Source: CAD feature listing. Evaluate the final solid. Frame: model axes, mm. A direction names the side the tool comes from. Round coordinates to 2 decimals unless told otherwise and drop trailing zeros. Write each loop counter-clockwise with the first axis right and the second up, starting at its lowest first coordinate (ties: lowest second). Pieces come first, ordered by that corner, then holes. Notation, with made-up numbers: M -20,-20.5 L 26,-20.5 A25 cw 26,4.5 Z; hole C 1.5,6 d4. An arc over 180 degrees is marked long. Put each result on its own line as item: value. Start each with the question number.
```python
from build123d import *

# Parameters (mm, degrees)
SKETCH8_W           = 50
SKETCH8_H           = 50
SKETCH9_W           = 50
SKETCH9_H           = 50
BOSS_EXTRUDE1_DEPTH = 110
SKETCH10_W          = 50
SKETCH10_H          = 400
BOSS_EXTRUDE2_DEPTH = 50
SKETCH11_W          = 50
SKETCH11_H          = 100
BOSS_EXTRUDE3_DEPTH = 10


with BuildPart() as part:
    # Sweep1: sweep along a path in Sketch1
    with BuildLine(Plane.XY) as sweep1_path:
        Line((-325, 200), (325, 200))
        Line((325, 200), (325, -200))
        Line((325, -200), (-325, -200))
    # Sketch8 → Sweep1 (sweep)
    with BuildSketch(Plane(origin=(0, 0, 0), x_dir=(0, 0, -1), z_dir=(1, 0, 0))):
        with Locations((25, 175)):
            Rectangle(SKETCH8_W, SKETCH8_H)
    sweep(path=sweep1_path.line, transition=Transition.RIGHT)

    # Sketch9 → Boss-Extrude1 (add)
    with BuildSketch(Plane.XY):
        with Locations((-300, 175)):
            Rectangle(SKETCH9_W, SKETCH9_H)
        with Locations((-300, -175)):
            Rectangle(SKETCH9_W, SKETCH9_H)
    extrude(amount=-BOSS_EXTRUDE1_DEPTH)

    # Sketch10 → Boss-Extrude2 (add)
    with BuildSketch(Plane.XY):
        with Locations((-50, 0)):
            Rectangle(SKETCH10_W, SKETCH10_H)
    extrude(amount=-BOSS_EXTRUDE2_DEPTH)

    # Sketch11 → Boss-Extrude3 (add)
    with BuildSketch(Plane(origin=(0, 0, -110), x_dir=(-1, 0, 0), z_dir=(0, 0, -1))):
        with Locations((300, 150)):
            Rectangle(SKETCH11_W, SKETCH11_H)
        with Locations((300, -150)):
            Rectangle(SKETCH11_W, SKETCH11_H)
    extrude(amount=-BOSS_EXTRUDE3_DEPTH)


solid = part.part
```
(1) Section query A-A (x = 164). Return loops of the section in (y, z), and give its area (3 significant figures).
(2) Pull-direction query (Y, two-part tool) for faces 1 (the flat face through (-5, -200, -30)), 2 (the flat face through (5, 200, -31)), 3 (the flat face through (275, -2, -25)), 4 (the flat face through (325, -3, -25)); classes: +Y half, -Y half, draft (parallel to the pull), parting line (faces both ways), or undercut.
(3) Section query B-B (y = 143.5). Return loops of the section in (x, z), and give its area (3 significant figures).
(4) Ray query, line 1 along Y through (x, z) = (57, -5); line 2 along Z through (x, y) = (-72, 147); line 3 along X through (y, z) = (156, -65.5). Return the intervals inside material, ascending.
(5) Section query C-C (z = -74). Return loops of the section in (x, y).
(6) Access query for faces 5 (the flat face through (-275, -173, -80)), 6 (the flat face through (-226, 150, -38)), 7 (the flat face through (-300, 125, -100)), 8 (the flat face through (127, 150, -25)). Directions: +Z, -Z, +X, -X, +Y, -Y. A direction counts if a zero-diameter tool reaches every point of the face in a straight line with its end or side. Return the directions, or none.
(7) Contact query for a flat-ended pin moving along its axis: P1, Ø15, axis at x = -310.5, y = -116.5, coming from the +Z side. Output: stop coordinate, or through.
(8) Section query D-D (z = -24.5). Return loops of the section in (x, y).
Entries:
1. outline: M -200,-50 L -150,-50 L -150,0 L -200,0 Z; M 150,-50 L 200,-50 L 200,0 L 150,0 Z
1. area: 5,000 mm2
2. face 1: -Y half
2. face 2: +Y half
2. face 3: undercut
2. face 4: draft
3. outline: M -325,-110 L -275,-110 L -275,-100 L -325,-100 Z; M -75,-50 L -25,-50 L -25,0 L -75,0 Z; M 275,-50 L 325,-50 L 325,0 L 275,0 Z
3. area: 5,500 mm2
4. line 1: -200 to -150, 150 to 200
4. line 2: -50 to 0
4. line 3: -325 to -275
5. outline: M -325,-200 L -275,-200 L -275,-150 L -325,-150 Z; M -325,150 L -275,150 L -275,200 L -325,200 Z
6. face 5: -Z, +X, +Y, -Y
6. face 6: +Z, -X
6. face 7: +Z, +X, -X
6. face 8: +Z, -Z
7. P1: z = -100
8. outline: M -325,-200 L 325,-200 L 325,200 L -325,200 L -325,150 L -75,150 L -75,-150 L -325,-150 Z; hole M -25,-150 L 275,-150 L 275,150 L -25,150 Z
